```python
from build123d import *

# Parameters (mm, degrees)
SKETCH_1_R      = 20.5
SKETCH_1_R_2    = 1.35
SKETCH_1_R_3    = 3.25
EXTRUDE_1_DEPTH = 4
SKETCH_1_3_R    = 3.25
SKETCH_1_3_R_2  = 1.5
EXTRUDE_2_DEPTH = 15
SKETCH_1_4_R    = 22.5
SKETCH_1_4_R_2  = 20.5
EXTRUDE_3_DEPTH = 20
FILLET_1_R      = 5
FILLET_2_R      = 2
CHAMFER_1_SIZE  = 1


with BuildPart() as part:
    # Sketch 1 → Extrude 1 (new body)
    with BuildSketch(Plane(origin=(0, 0, 0), x_dir=(1, 0, 0), z_dir=(0, 1, 0))):
        with Locations(Location((0, 0, 0), (0, 0, 270))):
            Circle(SKETCH_1_R)
        with Locations(Location((0, -7.75, 0), (0, 0, 270))):
            Circle(SKETCH_1_R_2, mode=Mode.SUBTRACT)
        with Locations(Location((7.75, 0, 0), (0, 0, 270))):
            Circle(SKETCH_1_R_2, mode=Mode.SUBTRACT)
        with Locations(Location((0, 7.75, 0), (0, 0, 270))):
            Circle(SKETCH_1_R_2, mode=Mode.SUBTRACT)
        with Locations(Location((-7.75, 0, 0), (0, 0, 270))):
            Circle(SKETCH_1_R_2, mode=Mode.SUBTRACT)
        with Locations(Location((0, 0, 0), (0, 0, 270))):
            Circle(SKETCH_1_R_3, mode=Mode.SUBTRACT)
        with BuildLine():
            ThreePointArc((4, -17.549928775), (12.727922061, -12.727922061), (17.549928775, -4))
            Line((17.549928775, -4), (4, -4))
            Line((4, -4), (4, -17.549928775))
        make_face(mode=Mode.SUBTRACT)
        with BuildLine():
            ThreePointArc((-17.549928775, -4), (-12.727922061, -12.727922061), (-4, -17.549928775))
            Line((-4, -17.549928775), (-4, -4))
            Line((-4, -4), (-17.549928775, -4))
        make_face(mode=Mode.SUBTRACT)
        with BuildLine():
            ThreePointArc((17.549928775, 4), (12.727922061, 12.727922061), (4, 17.549928775))
            Line((4, 17.549928775), (4, 4))
            Line((4, 4), (17.549928775, 4))
        make_face(mode=Mode.SUBTRACT)
        with BuildLine():
            ThreePointArc((-4, 17.549928775), (-12.727922061, 12.727922061), (-17.549928775, 4))
            Line((-17.549928775, 4), (-4, 4))
            Line((-4, 4), (-4, 17.549928775))
        make_face(mode=Mode.SUBTRACT)
    extrude(amount=EXTRUDE_1_DEPTH)

    # Sketch 1_3 → Extrude 2 (add)
    with BuildSketch(Plane(origin=(0, 0, 0), x_dir=(1, 0, 0), z_dir=(0, 1, 0))):
        with Locations(Location((0, 0, 0), (0, 0, 270))):
            Circle(SKETCH_1_3_R)
        with Locations(Location((0, 0, 0), (0, 0, 270))):
            Circle(SKETCH_1_3_R_2, mode=Mode.SUBTRACT)
    extrude(amount=EXTRUDE_2_DEPTH)

    # Sketch 1_4 → Extrude 3 (add)
    with BuildSketch(Plane(origin=(0, 0, 0), x_dir=(1, 0, 0), z_dir=(0, 1, 0))):
        with Locations(Location((0, 0, 0), (0, 0, 270))):
            Circle(SKETCH_1_4_R)
        with Locations(Location((0, 0, 0), (0, 0, 270))):
            Circle(SKETCH_1_4_R_2, mode=Mode.SUBTRACT)
    extrude(amount=EXTRUDE_3_DEPTH)

    # Fillet 1
    fillet_1_edges = [part.edges().sort_by_distance(p)[0] for p in [
        (-4, 2, -4),
        (4, 2, -4),
        (-4, 2, 4),
        (4, 2, 4),
    ]]
    fillet(fillet_1_edges, radius=FILLET_1_R)

    # Fillet 2
    fillet_2_edges = [part.edges().sort_by_distance(p)[0] for p in [
        (-17.549928775, 2, -4),
        (-4, 2, -17.549928775),
        (4, 2, -17.549928775),
        (17.549928775, 2, -4),
        (-4, 2, 17.549928775),
        (-17.549928775, 2, 4),
        (17.549928775, 2, 4),
        (4, 2, 17.549928775),
    ]]
    fillet(fillet_2_edges, radius=FILLET_2_R)

    # Chamfer 1
    chamfer_1_edges = [part.edges().sort_by_distance(p)[0] for p in [
        (0, 0, -22.5),
    ]]
    chamfer(chamfer_1_edges, length=CHAMFER_1_SIZE)


solid = part.part
```
Source: CAD feature listing. Evaluate the final solid. Frame: model axes, mm. A direction names the side the tool comes from. Round coordinates to 2 decimals unless told otherwise and drop trailing zeros. Write each loop counter-clockwise with the first axis right and the second up, starting at its lowest first coordinate (ties: lowest second). Pieces come first, ordered by that corner, then holes. Notation, with made-up numbers: M 44,19.25 L 89,19.25 A25 ccw 89,41.25 Z; hole C 39.25,14 d5. An arc over 180 degrees is marked long. Answer as a JSON object with one key per item and string values. Group by question number.
(1) First-contact query: pin 1 (2 mm diameter, centred on x = -11.5, y = 2.5, fed in from -Z); pin 2 (1 mm diameter, centred on x = -15.5, z = 10, fed in from +Y); pin 3 (1.2 mm diameter, centred on y = 2.5, z = 11, fed in from -X); pin 4 (2.5 mm diameter, centred on x = 0, z = 0, fed in from +Y). Flat tips, straight axial feed; report the tip coordinate or a pass-through.
(2) Section query D-D on y = 2.25. State how many separate pieces and enclosed holes the cut face has, then the cut area to 3 significant figures.
(3) Section query A-A on z = 0. Output: boundary loops of the cut face in (x, y).
(4) Section query B-B on y = 10. Output: boundary loops of the cut face in (x, z).
(5) Mould query, pull axis X, two halves, no side actions, for faces 3 (the flat face through (0, 0, 4)), 4 (the cylindrical face through (-8.618, 10.367, 20.784)), 5 (the flat face through (-12, 2, 4)). Classes: +X half, -X half, draft (parallel to the pull), parting line (faces both ways), or undercut.
(6) Ray query, line 1 (X direction, y = 2.15, z = 0); line 2 (X direction, y = 13, z = 0); line 3 (Y direction, x = -2.5, z = 3.5). Return the intervals inside material, ascending. Write a range as [from, to].
(7) Reachability of faces 1 (the flat face through (-9.9, 20, 18.2)), 2 (the flat face through (4, 2, -12)) from +Z, -Z, +X, -X, +Y, -Y: full face, straight path, thin tool, end or side. Return the list, or none.
(8) Section query C-C on x = 0. Output: boundary loops of the cut face in (y, z), then the cut area to 3 significant figures.
Computed values:
{
 "1": {"pin 1": "z = -19.9", "pin 2": "y = 4", "pin 3": "x = -19.95", "pin 4": "through"},
 "2": {"separate pieces": "1", "enclosed holes": "9", "area": "1,090 mm^2"},
 "3": {"outline": "M -22.5,1 L -21.5,0 L -9.1,0 L -9.1,4 L -20.5,4 L -20.5,20 L -22.5,20 Z; M -6.4,0 L -1.5,0 L -1.5,15 L -3.25,15 L -3.25,4 L -6.4,4 Z; M 1.5,0 L 6.4,0 L 6.4,4 L 3.25,4 L 3.25,15 L 1.5,15 Z; M 9.1,0 L 21.5,0 L 22.5,1 L 22.5,20 L 20.5,20 L 20.5,4 L 9.1,4 Z"},
 "4": {"outline": "C 0,0 d45; C 0,0 d6.5; hole C 0,0 d41; hole C 0,0 d3"},
 "5": {"face 3": "draft", "face 4": "parting line", "face 5": "undercut"},
 "6": {"line 1": "[-22.5, -9.1], [-6.4, -1.5], [1.5, 6.4], [9.1, 22.5]", "line 2": "[-22.5, -20.5], [-3.25, -1.5], [1.5, 3.25], [20.5, 22.5]", "line 3": "[0, 4]"},
 "7": {"face 1": "+Z, -Z, +X, -X, +Y", "face 2": "+Y, -Y"},
 "8": {"outline": "M 0,-21.5 L 1,-22.5 L 20,-22.5 L 20,-20.5 L 4,-20.5 L 4,-9.1 L 0,-9.1 Z; M 0,-6.4 L 4,-6.4 L 4,-3.25 L 15,-3.25 L 15,-1.5 L 0,-1.5 Z; M 0,1.5 L 15,1.5 L 15,3.25 L 4,3.25 L 4,6.4 L 0,6.4 Z; M 0,9.1 L 4,9.1 L 4,20.5 L 20,20.5 L 20,22.5 L 1,22.5 L 0,21.5 Z", "area": "248 mm^2"}
}
